Part model, mm, in its own coordinate system. A direction names the side the tool comes from. Coordinates: 2 decimals unless noted, no trailing zeros. Write each loop counter-clockwise with the first axis right and the second up, starting at its lowest first coordinate (ties: lowest second). Pieces come first, ordered by that corner, then holes. Notation, with made-up numbers: (76.25, -27.75) -> (98.25, -27.75) arc R16 ccw to (98.25, 1.25) -> close; hole circle Ø7 at (58.25, 22). An arc over 180 degrees is marked (long way). Write item = value, one per line. Start each with the question number.
Q1. Pull direction X, two halves, no side cores. Call faces 1 (the flat face through (-4, 0, -1052)), 2 (the flat face through (-274.12, 4.44, -1023.03)), 3 (the cylindrical face through (-0.1, 4.4, -1032.5)): released by +X, released by -X, zero draft, split by the parting line, or undercut.
Q2. Band-saw the part on A-A, the plane z = -1027. List the corners of the cut face in (x, y).
Q3. Band-saw the part on B-B, the plane y = 5.5. List the corners of the cut face in (x, z).
Q4. Band-saw the part on C-C, the plane x = -116.5. List the corners of the cut face in (y, z).
Q5. Band-saw the part on D-D, the plane x = 157.5. List the corners of the cut face in (y, z), plus the area to 3 significant figures.
Q6. Tool access for faces 4 (the cylindrical face through (-12.545, 4.563, -1032.786)), 5 (the cylindrical face through (3.977, 4.437, -1084.993)): list every direction of +Z, -Z, +X, -X, +Y, -Y with a clear straight run to the whole face (end or side of a thin tool).
Q7. Pin check, flat tips, straight feed: P1, Ø2, axis at x = -186, y = 6, coming from the -Z side; P2, Ø9, axis at x = -12.5, z = -1047.43, coming from the -Y side; P3, Ø1.5, axis at x = -206, y = 6.5, coming from the -Z side; P4, Ø1, axis at y = 6, z = -1010.5, coming from the +X side. Stop position of each tip, or through.
Q8. Probe line 1 (X direction, y = 3.25, z = -1044); line 2 (X direction, y = 1, z = -1048); line 3 (X direction, y = 6.5, z = -1018). List the from-to ranges inside material, lowest first.
from build123d import *

# Parameters (mm, degrees)
SKETCH1_R           = 4
BOSS_EXTRUDE1_DEPTH = 9
FILLET1_R           = 30


with BuildPart() as part:
    # Sketch1 → Boss-Extrude1 (new body)
    with BuildSketch(Plane(origin=(0, 0, 0), x_dir=(1, 0, 0), z_dir=(0, 1, 0))):
        with BuildLine():
            ThreePointArc((-267.230664068, 997.318415643), (-261.188620877, 998.917791575), (-255.137006757, 1000.480563421))
            Line((-255.137006757, 1000.480563421), (-231.630657469, 1019.00551447))
            ThreePointArc((-231.630657469, 1019.00551447), (-141.360133679, 1035.394761724), (-50, 1043.80314236))
            Line((-50, 1043.80314236), (-12.5, 1032.424331368))
            ThreePointArc((-12.5, 1032.424331368), (0, 1032.5), (12.5, 1032.424331368))
            Line((12.5, 1032.424331368), (50, 1043.80314236))
            ThreePointArc((50, 1043.80314236), (141.360133679, 1035.394761724), (231.630657469, 1019.00551447))
            Line((231.630657469, 1019.00551447), (255.137006757, 1000.480563421))
            ThreePointArc((255.137006757, 1000.480563421), (261.188620877, 998.917791575), (267.230664068, 997.318415643))
            Line((267.230664068, 997.318415643), (280.818663936, 1048.029521524))
            ThreePointArc((280.818663936, 1048.029521524), (0, 1085), (-280.818663936, 1048.029521524))
            Line((-280.818663936, 1048.029521524), (-267.230664068, 997.318415643))
        make_face()
        with Locations(Location((-12.5, 1047.425415006, 0), (0, 0, 270))):
            Circle(SKETCH1_R, mode=Mode.SUBTRACT)
        with Locations(Location((12.5, 1047.425415006, 0), (0, 0, 270))):
            Circle(SKETCH1_R, mode=Mode.SUBTRACT)
        with Locations(Location((-259.019572899, 1014.970497529, 0), (0, 0, 270))):
            Circle(SKETCH1_R, mode=Mode.SUBTRACT)
        with Locations(Location((259.019572899, 1014.970497529, 0), (0, 0, 270))):
            Circle(SKETCH1_R, mode=Mode.SUBTRACT)
    extrude(amount=BOSS_EXTRUDE1_DEPTH)

    # Fillet1
    fillet1_edges = [part.edges().sort_by_distance(p)[0] for p in [
        (50, 4.5, -1043.80314236),
        (12.5, 4.5, -1032.424331368),
        (-12.5, 4.5, -1032.424331368),
        (-50, 4.5, -1043.80314236),
        (-231.630657469, 4.5, -1019.00551447),
        (-255.137006757, 4.5, -1000.480563421),
        (255.137006757, 4.5, -1000.480563421),
        (231.630657469, 4.5, -1019.00551447),
    ]]
    fillet(fillet1_edges, radius=FILLET1_R)


solid = part.part
Ans:
q1.face_1 = zero draft
q1.face_2 = released by -X
q1.face_3 = undercut
q2.outline = (-275.18, 0) -> (-193.12, 0) -> (-193.12, 9) -> (-275.18, 9) -> close; (193.12, 0) -> (275.18, 0) -> (275.18, 9) -> (193.12, 9) -> close
q3.outline = (-280.82, -1048.03) arc R1085 ccw to (280.82, -1048.03) -> (267.23, -997.32) arc R1032.5 cw to (261.16, -998.93) arc R30 ccw to (250.18, -1004.39) -> (236.99, -1014.78) arc R30 cw to (224.88, -1020.52) arc R1045 cw to (55.3, -1043.54) arc R30 cw to (45, -1042.29) -> (16.9, -1033.76) arc R30 ccw to (7.96, -1032.47) arc R1032.5 cw to (-7.96, -1032.47) arc R30 ccw to (-16.9, -1033.76) -> (-45, -1042.29) arc R30 cw to (-55.3, -1043.54) arc R1045 cw to (-224.88, -1020.52) arc R30 cw to (-236.99, -1014.78) -> (-250.18, -1004.39) arc R30 ccw to (-261.16, -998.93) arc R1032.5 cw to (-267.23, -997.32) -> close; hole circle Ø8 at (-259.02, -1014.97); hole circle Ø8 at (-12.5, -1047.43); hole circle Ø8 at (12.5, -1047.43); hole circle Ø8 at (259.02, -1014.97)
q4.outline = (0, -1078.73) -> (9, -1078.73) -> (9, -1038.49) -> (0, -1038.49) -> close
q5.outline = (0, -1073.51) -> (9, -1073.51) -> (9, -1033.06) -> (0, -1033.06) -> close
q5.area = 364 mm2
q6.face_4 = +Z, +Y, -Y
q6.face_5 = -Z, +Y, -Y
q7.P1 = -1069.11
q7.P2 = 0
q7.P3 = -1065.41
q7.P4 = 270.9
q8.line_1 = -279.74 to -14.57, -10.43 to 10.43, 14.57 to 279.74
q8.line_2 = -280.81 to -16.46, -8.54 to 8.54, 16.46 to 280.81
q8.line_3 = -272.77 to -261.63, -256.41 to -231.94, 231.94 to 256.41, 261.63 to 272.77
